```python
from build123d import *

# Parameters (mm, degrees)
BOSS_EXTRUDE1_DEPTH     = 15
CUT_EXTRUDE1_DEPTH      = 107.066017202
CUT_EXTRUDE1_DEPTH_BACK = 107.066017202
SKETCH8_R               = 7.5
CUT_EXTRUDE2_DEPTH      = 98.596106557
CUT_EXTRUDE2_DEPTH_BACK = 8
SKETCH9_R               = 0.75
SKETCH9_R_2             = 3


with BuildPart() as part:
    # Sketch1 → Revolve1 (revolve)
    with BuildSketch(Plane(origin=(0, 0, 0), x_dir=(0, 0, -1), z_dir=(1, 0, 0)), mode=Mode.PRIVATE) as revolve1_sk:
        Polygon((0, 0), (-40, 0), (-40, 15), (-20, 15), (-20, 25), (20, 25), (20, 15), (40, 15), (40, 0), align=None)
    revolve(revolve1_sk.sketch.rotate(Axis((0, 0, 74.697986577), (0, 0, -1)), 90), axis=Axis((0, 0, 74.697986577), (0, 0, -1)))

    # Sketch3 → Loft1 section 0
    with BuildSketch(Plane(origin=(-50, 0, 0), x_dir=(0, 0, -1), z_dir=(1, 0, 0))):
        with BuildLine():
            Line((-10, 10), (10, 10))
            Line((10, 10), (10, -10))
            Line((10, -10), (-10, -10))
            Line((-10, -10), (-10, 10))
        make_face()
    # Sketch4 → Loft1 section 1
    with BuildSketch(Plane(origin=(30, 0, 0), x_dir=(0, 0, -1), z_dir=(1, 0, 0))):
        with BuildLine():
            Line((-15, 15), (15, 15))
            Line((15, 15), (15, -15))
            Line((15, -15), (-15, -15))
            Line((-15, -15), (-15, 15))
        make_face()
    loft()

    # Sketch7 → Boss-Extrude1 (add, symmetric)
    with BuildSketch(Plane.XY):
        with BuildLine():
            Line((30, 15), (30, -15))
            ThreePointArc((30, -15), (45, 0), (30, 15))
        make_face()
    extrude(amount=BOSS_EXTRUDE1_DEPTH, both=True)

    # Sketch8 → Cut-Extrude1 (cut, two sides: drawn at the far end of the back side and taken through both)
    with BuildSketch(Plane.ZY.offset(50).offset(-CUT_EXTRUDE1_DEPTH_BACK)):
        Circle(SKETCH8_R)
    extrude(amount=CUT_EXTRUDE1_DEPTH + CUT_EXTRUDE1_DEPTH_BACK, mode=Mode.SUBTRACT)

    # Sketch9 → Cut-Extrude2 (cut, two sides: drawn at the far end of the back side and taken through both)
    with BuildSketch(Plane(origin=(0, 0, -40), x_dir=(-1, 0, 0), z_dir=(0, 0, -1)).offset(-CUT_EXTRUDE2_DEPTH_BACK)):
        with Locations(Location((0, 7.2, 0), (0, 0, 180))):
            Circle(SKETCH9_R)
        with Locations(Location((0, 10.4, 0), (0, 0, 180))):
            Circle(SKETCH9_R)
        with Locations(Location((0, 13.6, 0), (0, 0, 180))):
            Circle(SKETCH9_R)
        with Locations(Location((11.777945491, 6.8, 0), (0, 0, 180))):
            Circle(SKETCH9_R)
        with Locations(Location((9.006664199, 5.2, 0), (0, 0, 180))):
            Circle(SKETCH9_R)
        with Locations(Location((6.235382907, 3.6, 0), (0, 0, 180))):
            Circle(SKETCH9_R)
        with Locations(Location((11.777945491, -6.8, 0), (0, 0, 180))):
            Circle(SKETCH9_R)
        with Locations(Location((9.006664199, -5.2, 0), (0, 0, 180))):
            Circle(SKETCH9_R)
        with Locations(Location((6.235382907, -3.6, 0), (0, 0, 180))):
            Circle(SKETCH9_R)
        with Locations(Location((0, -13.6, 0), (0, 0, 180))):
            Circle(SKETCH9_R)
        with Locations(Location((0, -10.4, 0), (0, 0, 180))):
            Circle(SKETCH9_R)
        with Locations(Location((0, -7.2, 0), (0, 0, 180))):
            Circle(SKETCH9_R)
        with Locations(Location((-11.777945491, -6.8, 0), (0, 0, 180))):
            Circle(SKETCH9_R)
        with Locations(Location((-9.006664199, -5.2, 0), (0, 0, 180))):
            Circle(SKETCH9_R)
        with Locations(Location((-6.235382907, -3.6, 0), (0, 0, 180))):
            Circle(SKETCH9_R)
        with Locations(Location((-11.777945491, 6.8, 0), (0, 0, 180))):
            Circle(SKETCH9_R)
        with Locations(Location((-9.006664199, 5.2, 0), (0, 0, 180))):
            Circle(SKETCH9_R)
        with Locations(Location((-6.235382907, 3.6, 0), (0, 0, 180))):
            Circle(SKETCH9_R)
        with Locations(Location((0, 0, 0), (0, 0, 180))):
            Circle(SKETCH9_R_2)
    extrude(amount=CUT_EXTRUDE2_DEPTH + CUT_EXTRUDE2_DEPTH_BACK, mode=Mode.SUBTRACT)


solid = part.part
```
Geometry: final body of the model. Coordinates: model frame, mm. A direction names the side the tool comes from. Round coordinates to 2 decimals unless told otherwise and drop trailing zeros. Order: outer loops, then holes, each group sorted by start corner. A loop starts at its lowest first (then second) coordinate and runs counter-clockwise, first axis right, second up. Notation, with made-up numbers: M -17.75,62 L 4.25,62 A13 cw 4.25,69 Z; hole C 44,-23 d7. An arc over 180 degrees is marked long. Use one line per item in the form item = value. Start each with the question number.
Q1. Cut plane A-A (z = -16.5). Return loops of the section in (x, y), and give its area (3 significant figures).
Q2. Pin query (flat end, axial travel): pin 1 Ø8 at (x, z) = (27, 6) entering from -Y; pin 2 Ø4 at (x, z) = (4, -1.5) entering from +Y; pin 3 Ø8 at (x, z) = (-19, -12) entering from +Y. Return the tip coordinate at first contact, or that it passes through.
Q3. Cut plane B-B (y = -18.5). Return loops of the section in (x, z), and give its area (3 significant figures).
Q4. Mould query, pull axis Y, two halves, no side actions, for faces 6 (the face through (-20, 15, 0)), 7 (the face through (-4, 0, -40)), 8 (the face through (2.86, -0.9, -35.94)). Classes: +Y half, -Y half, draft (parallel to the pull), parting line (faces both ways), or undercut.
Q5. Access query for faces 1 (the face through (36, 0, 15)), 2 (the face through (0, 0, -32)), 3 (the face through (8.06, -12.65, 29.86)), 4 (the face through (36, 0, -15)), 5 (the face through (0, 0, 40)). Directions: +Z, -Z, +X, -X, +Y, -Y. A direction counts if a zero-diameter tool reaches every point of the face in a straight line with its end or side. Return the directions, or none.
Q6. Cut plane C-C (z = 26). Return loops of the section in (x, y), and give its area (3 significant figures).
Q7. Material intervals for line 1 (Z direction, x = -11.5, y = -0.5); line 2 (X direction, y = 7.2, z = -34.5); line 3 (Z direction, x = -24.5, y = 0), sorted ascending. Write a range as [from, to].
Geometry results:
q1.outline = C 0,0 d50
q1.area = 1,960 mm^2
q2.pin_1 = -15
q2.pin_2 = 24.92
q2.pin_3 = 20
q3.outline = M -16.82,-20 L 16.82,-20 L 16.82,20 L -16.82,20 Z
q3.area = 1,350 mm^2
q4.face_6 = parting line
q4.face_7 = draft
q4.face_8 = undercut
q5.face_1 = +Z, +X, +Y, -Y
q5.face_2 = -Z
q5.face_3 = +Z
q5.face_4 = -Z, +X, +Y, -Y
q5.face_5 = +Z, +X, -X, +Y, -Y
q6.outline = C 0,0 d30
q6.area = 707 mm^2
q7.line_1 = [-40, -7.48], [7.48, 40]
q7.line_2 = [-13.16, -12.41], [-11.14, -0.75], [0.75, 11.14], [12.41, 13.16]
q7.line_3 = [-20, -7.5], [7.5, 20]
